```python
from build123d import *

# Parameters (mm, degrees)
BASE_FLANGE1_START           = -0.5
BASE_FLANGE1_OUTLINE_W       = 91
BASE_FLANGE1_OUTLINE_H       = 75
BASE_FLANGE1_DEPTH           = 1
EDGE_FLANGE1_STRIP_W         = 8
EDGE_FLANGE1_STRIP_H         = 1
EDGE_FLANGE1_STRIP_CUT_DEPTH = 75
EDGE_FLANGE1_DEPTH           = 75
EDGE_FLANGE2_STRIP_W         = 14
EDGE_FLANGE2_STRIP_H         = 1
EDGE_FLANGE2_STRIP_CUT_DEPTH = 75
EDGE_FLANGE2_DEPTH           = 75
EDGE_FLANGE3_START           = -42.5
EDGE_FLANGE3_DEPTH           = 85
EDGE_FLANGE3_2_DEPTH         = 85
CUT_EXTRUDE1_DEPTH           = 111.402059319
CUT_EXTRUDE1_DEPTH_BACK      = 111.402059319
CUT_EXTRUDE2_DEPTH           = 114.152126139
CUT_EXTRUDE2_DEPTH_BACK      = 114.152126139
SKETCH16_R                   = 7.5


# Read off the part's stored shape, not the designer's step: Base-Flange1, Edge-Flange3
# Sheet-metal steps are written as plain solids
with BuildPart() as part:
    # Base-Flange1 outline → Base-Flange1 (new body)
    with BuildSketch(Plane(origin=(0, 0, 0), x_dir=(0, 1, 0), z_dir=(0, 0, 1)).offset(BASE_FLANGE1_START)):
        Rectangle(BASE_FLANGE1_OUTLINE_W, BASE_FLANGE1_OUTLINE_H)
    extrude(amount=BASE_FLANGE1_DEPTH)

    # Edge-Flange1 strip (across the edge) → Edge-Flange1 strip cut (cut)
    with BuildSketch(Plane(origin=(37.5, -45.5, -0.5), x_dir=(0, 1, 0), z_dir=(-1, 0, 0))):
        with Locations((-1, -0.5)):
            Rectangle(EDGE_FLANGE1_STRIP_W, EDGE_FLANGE1_STRIP_H)
    edge_flange1_strip_cut = extrude(amount=EDGE_FLANGE1_STRIP_CUT_DEPTH, mode=Mode.SUBTRACT)

    # Edge-Flange1 section (across the edge) → Edge-Flange1 (add)
    with BuildSketch(Plane(origin=(37.5, -45.5, -0.5), x_dir=(0, 1, 0), z_dir=(-1, 0, 0))):
        with BuildLine():
            Line((0, 2), (0, 19))
            Line((0, 19), (1, 19))
            Line((1, 19), (1, 2))
            ThreePointArc((1, 2), (1.585786438, 0.585786438), (3, 0))
            Line((3, 0), (3, -1))
            ThreePointArc((3, -1), (0.878679656, -0.121320344), (0, 2))
        make_face()
    edge_flange1 = extrude(amount=EDGE_FLANGE1_DEPTH)

    # Edge-Flange2 strip (across the edge) → Edge-Flange2 strip cut (cut)
    with BuildSketch(Plane(origin=(-37.5, -45.5, -19.5), x_dir=(0, 0, 1), z_dir=(1, 0, 0))):
        with Locations((-1, -0.5)):
            Rectangle(EDGE_FLANGE2_STRIP_W, EDGE_FLANGE2_STRIP_H)
    edge_flange2_strip_cut = extrude(amount=EDGE_FLANGE2_STRIP_CUT_DEPTH, mode=Mode.SUBTRACT)

    # Edge-Flange2 section (across the edge) → Edge-Flange2 (add)
    with BuildSketch(Plane(origin=(-37.5, -45.5, -19.5), x_dir=(0, 0, 1), z_dir=(1, 0, 0))):
        with BuildLine():
            Line((0, 5), (0, 49))
            Line((0, 49), (1, 49))
            Line((1, 49), (1, 5))
            ThreePointArc((1, 5), (2.464466094, 1.464466094), (6, 0))
            Line((6, 0), (6, -1))
            ThreePointArc((6, -1), (1.757359313, 0.757359313), (0, 5))
        make_face()
    edge_flange2 = extrude(amount=EDGE_FLANGE2_DEPTH)

    # Mirror1: Edge-Flange1 strip cut, Edge-Flange1, Edge-Flange2 strip cut, Edge-Flange2 across plane
    add(edge_flange1_strip_cut.mirror(Plane.ZX), mode=Mode.SUBTRACT)
    add(edge_flange1.mirror(Plane.ZX))
    add(edge_flange2_strip_cut.mirror(Plane.ZX), mode=Mode.SUBTRACT)
    add(edge_flange2.mirror(Plane.ZX))

    # Edge-Flange3 outline → Edge-Flange3 (cut)
    with BuildSketch(Plane(origin=(0, 0, 0), x_dir=(1, 0, 0), z_dir=(0, 1, 0)).offset(EDGE_FLANGE3_START)):
        with BuildLine():
            ThreePointArc((36.044119063, 0.5), (36.780075537, 0.44554022), (37.5, 0.283347228))
            Line((37.5, 0.283347228), (37.5, 0.5))
            Line((37.5, 0.5), (36.044119063, 0.5))
        make_face()
    edge_flange3 = extrude(amount=EDGE_FLANGE3_DEPTH, mode=Mode.SUBTRACT)

    # Edge-Flange3 2 outline → Edge-Flange3 2 (add)
    with BuildSketch(Plane(origin=(0, 0, 0), x_dir=(1, 0, 0), z_dir=(0, 1, 0)).offset(EDGE_FLANGE3_START)):
        with BuildLine():
            Line((53.463676472, -12.589707751), (39.258057111, -0.669777784))
            ThreePointArc((39.258057111, -0.669777784), (38.427166306, -0.104424288), (37.5, 0.283347228))
            Line((37.5, 0.283347228), (37.5, -0.5))
            Line((37.5, -0.5), (36.044119063, -0.5))
            ThreePointArc((36.044119063, -0.5), (37.412199636, -0.741229517), (38.615269502, -1.435822228))
            Line((38.615269502, -1.435822228), (52.820888862, -13.355752194))
            Line((52.820888862, -13.355752194), (53.463676472, -12.589707751))
        make_face()
    edge_flange3_2 = extrude(amount=EDGE_FLANGE3_2_DEPTH)

    # Mirror2: Edge-Flange3, Edge-Flange3 2 across plane
    add(edge_flange3.mirror(Plane(origin=(0, 0, 0), x_dir=(0, 0, 1), z_dir=(1, 0, 0))), mode=Mode.SUBTRACT)
    add(edge_flange3_2.mirror(Plane(origin=(0, 0, 0), x_dir=(0, 0, 1), z_dir=(1, 0, 0))))

    # Sketch15 → Cut-Extrude1 (cut, two sides: drawn at the far end of the back side and taken through both)
    with BuildSketch(Plane.XY.offset(0.5).offset(-CUT_EXTRUDE1_DEPTH_BACK)):
        with BuildLine():
            Line((-26.955880937, 5), (-14.955880937, 5))
            ThreePointArc((-14.955880937, 5), (-9.955880937, 0), (-14.955880937, -5))
            Line((-14.955880937, -5), (-26.955880937, -5))
            ThreePointArc((-26.955880937, -5), (-31.955880937, 0), (-26.955880937, 5))
        make_face()
        with BuildLine():
            Line((17.262112136, 19.898855266), (11.262112136, 9.50655042))
            ThreePointArc((11.262112136, 9.50655042), (4.431985117, 7.676423401), (2.601858098, 14.50655042))
            Line((2.601858098, 14.50655042), (8.601858098, 24.898855266))
            ThreePointArc((8.601858098, 24.898855266), (15.431985117, 26.728982285), (17.262112136, 19.898855266))
        make_face()
        with BuildLine():
            Line((8.055902747, -25.844477673), (2.055902747, -15.452172827))
            ThreePointArc((2.055902747, -15.452172827), (3.886029766, -8.622045809), (10.716156785, -10.452172827))
            Line((10.716156785, -10.452172827), (16.716156785, -20.844477673))
            ThreePointArc((16.716156785, -20.844477673), (14.886029766, -27.674604692), (8.055902747, -25.844477673))
        make_face()
    extrude(amount=CUT_EXTRUDE1_DEPTH + CUT_EXTRUDE1_DEPTH_BACK, mode=Mode.SUBTRACT)

    # Sketch16 → Cut-Extrude2 (cut, two sides: drawn at the far end of the back side and taken through both)
    with BuildSketch(Plane.XY.offset(-18.5).offset(-CUT_EXTRUDE2_DEPTH_BACK)):
        with Locations((-17.5, 65.5)):
            Circle(SKETCH16_R)
        with Locations(Location((-17.5, -65.5, 0), (0, 0, 270))):
            Circle(SKETCH16_R)
    extrude(amount=CUT_EXTRUDE2_DEPTH + CUT_EXTRUDE2_DEPTH_BACK, mode=Mode.SUBTRACT)


solid = part.part
```
Could you check a few things on this model? Use its own coordinates, in mm. A direction names the side the tool comes from. Coordinates: 2 decimals unless noted, no trailing zeros. Loops run counter-clockwise (first coordinate to the right, second up) from the corner with the lowest first, then second, coordinate; pieces in that order, holes last.
1) Which directions (+Z, -Z, +X, -X, +Y, -Y) give clear straight access to the entire face, cutting with the end or side of a thin tool? Please do faces 5 (the face through (1, 44.5, -8)), 6 (the face through (-9.957, 0.11, -0.007)), 7 (the face through (-1, -72, -19.5)).
Reported:
face 5: -Z, +X, -X
face 6: +Z, -Z
face 7: -Z, +X, -X, +Y, -Y
2) Thinking about a two-plate mould opening in X: for faces 1 (the face through (46.46, -0.595, 6.713)), 2 (the face through (-37.5, 65, -19)), 3 (the face through (1, -44.5, -8)), 4 (the face through (-45.619, -0.595, 7.312)), which applies, released by +X, released by -X, zero draft, split by the parting line, or undercut?
Reported:
face 1: released by +X
face 2: released by -X
face 3: zero draft
face 4: undercut
3) Imagine slicing it at B-B (x = -17.5). State how many separate pieces and enclosed holes the cut face has, and give its area (3 significant figures).
Reported:
separate pieces: 4
enclosed holes: 0
area: 180 mm2
4) Imagine slicing it at D-D (y = -65.5). List the corners of the cut face in (x, z) for me.
Reported:
outline: (-37.5, -19.5) - (-25, -19.5) - (-25, -18.5) - (-37.5, -18.5) - close; (-10, -19.5) - (37.5, -19.5) - (37.5, -18.5) - (-10, -18.5) - close
5) Please list where these lines run through material, in increasing order: line 1 along X through (y, z) = (65, -19); line 2 along Z through (x, y) = (-27, -35); line 3 along Y through (x, z) = (-15, -17.5).
Reported:
line 1: x = -37.5 to -24.98, -10.02 to 37.5
line 2: z = -0.5 to 0.5
line 3: y = -47.5 to -46.03, 46.03 to 47.5
6) Will these pins go through, and if not, where does the flat tip stop? pin 1 Ø4 at (x, y) = (4.5, -6.5) entering from +Z; pin 2 Ø10 at (x, y) = (-8, 64.5) entering from +Z; pin 3 Ø9 at (x, z) = (-14.5, -10.5) entering from -Y.
Reported:
pin 1: stops at z = 0.5
pin 2: stops at z = -18.5
pin 3: stops at y = -45.73
7) Imagine slicing it at A-A (z = 9). List the corners of the cut face in (x, y) for me, and give its area (3 significant figures).
Reported:
outline: (-49.19, -42.5) - (-47.63, -42.5) - (-47.63, 42.5) - (-49.19, 42.5) - close; (47.63, -42.5) - (49.19, -42.5) - (49.19, 42.5) - (47.63, 42.5) - close
area: 264 mm2
8) Imagine slicing it at C-C (y = 0). List the corners of the cut face in (x, z) for me.
Reported:
outline: (-53.46, 12.59) - (-39.26, 0.67) arc R5 ccw to (-36.04, -0.5) - (-31.96, -0.5) - (-31.96, 0.5) - (-36.04, 0.5) arc R4 cw to (-38.62, 1.44) - (-52.82, 13.36) - close; (-9.96, -0.5) - (36.04, -0.5) arc R5 ccw to (39.26, 0.67) - (53.46, 12.59) - (52.82, 13.36) - (38.62, 1.44) arc R4 cw to (36.04, 0.5) - (-9.96, 0.5) - close
